Could you check a few things on this model? Use its own coordinates, in mm. Round coordinates to 2 decimals unless told otherwise and drop trailing zeros. Loops run counter-clockwise (first coordinate to the right, second up) from the corner with the lowest first, then second, coordinate; pieces in that order, holes last. Notation, with made-up numbers: (18.5, 7) -> (59.5, 7) arc R4 cw to (59.5, 12) -> close; hole circle Ø6 at (15.25, -0.75). An arc over 180 degrees is marked (long way). Write each question's results on one line, items separated by ' | '. Start each with the question number.
1) Imagine slicing it at C-C, the plane y = -6.5. List the corners of the cut face in (x, z) for me.
2) For P1, Ø3, axis at x = -2.5, y = 9.5, coming from the +Z side; P2, Ø1.5, axis at y = -5, z = 1.5, coming from the +X side; P3, Ø1.5, axis at y = -8.5, z = -3, coming from the -X side, each with a flat end and sliding along its axis, tell me the tip position at first contact or that it passes through.
3) We'd pull the mould along Y, two halves only. Please class faces 1 (the cylindrical face through (-0.945, -0.724, 14.858)), 2 (the flat face through (-4, 12.665, -13)), 3 (the flat face through (-4, -12.656, -13)): pulls with the +Y half, pulls with the -Y half, needs draft (parallel to the pull), parting line crosses it, or undercut.
4) Imagine slicing it at A-A, the plane z = 0. List the corners of the cut face in (x, y) for me (1 decimal), plus the area to 3 significant figures.
5) Imagine slicing it at D-D, the plane z = 15. List the corners of the cut face in (x, y) for me (3 decimals), plus the area to 3 significant figures.
6) If I drill on probe 1 along Z at (x, y) = (-0.5, 8.25); probe 2 along Y at (x, z) = (0, 15) (3 decimals); probe 3 along Z at (x, y) = (2, 3.5), over which ranges is the centre line in solid material (lowest first)?
7) Imagine slicing it at B-B, the plane x = 0. List the corners of the cut face in (y, z) for me (1 decimal).
from build123d import *

# Parameters (mm, degrees)
F2_R          = 17.199
F2_R_2        = 12.6365
F3_DEPTH      = 12.665
F3_DEPTH_BACK = 12.656
F5_R          = 1.190625
F6_DEPTH      = 17.2


with BuildPart() as f1:
    # F0 (on Top) → F1 (revolve)
    with BuildSketch(Plane.XY):
        with BuildLine():
            Line((13.1365, 12.665), (17.399, 12.665))
            Line((17.399, 12.665), (17.399, 14.165))
            Line((17.399, 14.165), (11.1365, 14.165))
            Line((11.1365, 14.165), (11.1365, -14.156))
            Line((11.1365, -14.156), (17.399, -14.156))
            Line((17.399, -14.156), (17.399, -12.656))
            Line((17.399, -12.656), (13.1365, -12.656))
            ThreePointArc((13.1365, -12.656), (12.7829466094, -12.5095533906), (12.6365, -12.156))
            Line((12.6365, -12.156), (12.6365, 12.165))
            ThreePointArc((12.6365, 12.165), (12.7829466094, 12.5185533906), (13.1365, 12.665))
        make_face()
    revolve(axis=Axis((0, 2.8540128842, 0), (0, 1, 0)))


with BuildPart() as f3:
    # F2 (on Front) → F3 (new body, two sides)
    with BuildSketch(Plane.XZ) as f3_sk:
        Circle(F2_R)
        Circle(F2_R_2, mode=Mode.SUBTRACT)
    extrude(amount=-F3_DEPTH)
    extrude(f3_sk.sketch, amount=F3_DEPTH_BACK)

    # F4: cut F1
    add(f1.part, mode=Mode.SUBTRACT)

    # F5 (on Top) → F6 (cut, through all)
    with BuildSketch(Plane.XY):
        Circle(F5_R)
    extrude(amount=F6_DEPTH, mode=Mode.SUBTRACT)


solid = f3.part
Checked values:
1) outline: circle Ø34.4 at (0, 0); hole circle Ø25.27 at (0, 0)
2) P1: z = 17.17 | P2: x = 17.18 | P3: x = -17.05
3) face 1: undercut | face 2: pulls with the +Y half | face 3: pulls with the -Y half
4) outline: (-17.2, -12.7) -> (-13.1, -12.7) arc R0.5 ccw to (-12.6, -12.2) -> (-12.6, 12.2) arc R0.5 ccw to (-13.1, 12.7) -> (-17.2, 12.7) -> close; (12.6, -12.2) arc R0.5 ccw to (13.1, -12.7) -> (17.2, -12.7) -> (17.2, 12.7) -> (13.1, 12.7) arc R0.5 ccw to (12.6, 12.2) -> close | area: 231 mm^2
5) outline: (-8.415, -12.656) -> (8.415, -12.656) -> (8.415, 12.665) -> (-8.415, 12.665) -> close; hole circle Ø2.381 at (0, 0) | area: 422 mm^2
6) probe 1: -17.19 to -12.63, 12.63 to 17.19 | probe 2: -12.656 to -1.191, 1.191 to 12.665 | probe 3: -17.08 to -12.48, 12.48 to 17.08
7) outline: (-12.7, -17.2) -> (12.7, -17.2) -> (12.7, -13.1) arc R0.5 ccw to (12.2, -12.6) -> (-12.2, -12.6) arc R0.5 ccw to (-12.7, -13.1) -> close; (-12.7, 13.1) arc R0.5 ccw to (-12.2, 12.6) -> (-1.2, 12.6) -> (-1.2, 17.2) -> (-12.7, 17.2) -> close; (1.2, 12.6) -> (12.2, 12.6) arc R0.5 ccw to (12.7, 13.1) -> (12.7, 17.2) -> (1.2, 17.2) -> close
